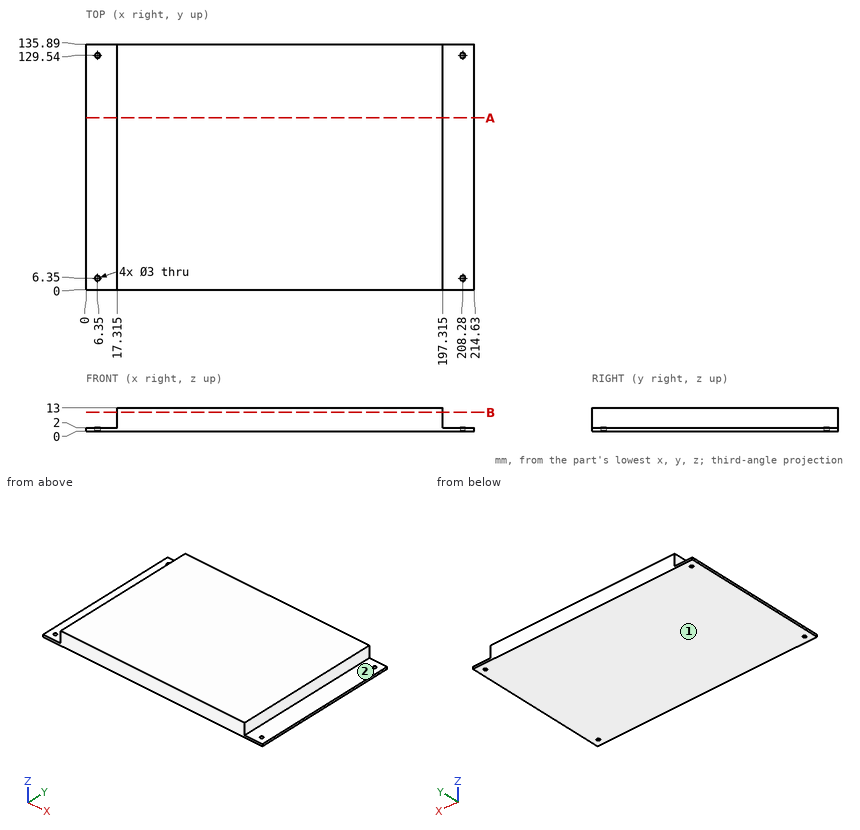
Answer from the drawing. Dimensions are ordinates in mm from the lowest x, y and z of the part. A direction names the side the tool comes from. Give positions to 0.01 mm unless a question says otherwise; leave off trailing zeros. Loops run counter-clockwise (first coordinate to the right, second up) from the corner with the lowest first, then second, coordinate; pieces in that order, holes last. Notation, with made-up numbers: (53.25, 52) -> (98.25, 52) arc R26 cw to (98.25, 67) -> close; hole circle Ø7 at (-39, 50.5). An arc over 180 degrees is marked (long way). One line per question, with ' | ' between items. Start each with the question number.
1) Section A-A, the plane y = 95 is taken. Determine the outline of the cut face in (x, z) (3 decimals), then the cut area to 3 significant figures.
2) Straight lines are drawn through the part: L1, parallel to X at y = 129.54, z = 1.2; L2, parallel to Y at x = 208.28, z = 0.5; L3, parallel to X at y = 53, z = 4.5 (3 decimals). For each, find the intervals that lie inside material, in ascending order.
3) Section B-B, the plane z = 10.5 is taken. Determine the outline of the cut face in (x, y) (3 decimals), then the cut area to 3 significant figures.
4) Each of these flat-tipped pins is pushed along its axis until it touches: pin 1 (4 mm diameter, centred on y = 62, z = 11.5, fed in from +X) (3 decimals); pin 2 (5 mm diameter, centred on x = 210, y = 76.5, fed in from +Z); pin 3 (2.5 mm diameter, centred on x = 6.35, y = 6.35, fed in from -Z). Where does it stop, or does it pass through?
5) For the marked faces 1 and 2, determine the directions among +Z, -Z, +X, -X, +Y, -Y from which every point of the face is accessible in a straight line to the end or side of a thin tool.
Resolved:
1) outline: (0, 0) -> (214.63, 0) -> (214.63, 2) -> (197.315, 2) -> (197.315, 13) -> (17.315, 13) -> (17.315, 2) -> (0, 2) -> close | area: 2,410 mm2
2) L1: 0 to 4.85, 7.85 to 206.78, 209.78 to 214.63 | L2: 0 to 4.85, 7.85 to 128.04, 131.04 to 135.89 | L3: 17.315 to 197.315
3) outline: (17.315, 0) -> (197.315, 0) -> (197.315, 135.89) -> (17.315, 135.89) -> close | area: 24,500 mm2
4) pin 1: x = 197.315 | pin 2: z = 2 | pin 3: through
5) face 1: -Z, +X, -X, +Y, -Y | face 2: +Z, +X, +Y, -Y
